```python
from build123d import *
from build123d.topology import SkipClean

# Parameters (mm, degrees)
SKETCH1_W           = 5.06
SKETCH1_H           = 1.900618781
FILLET1_R           = 1
SKETCH2_R           = 7.5
BOSS_EXTRUDE1_DEPTH = 20
SKETCH3_R           = 5.06
CUT_EXTRUDE1_DEPTH  = 5
SKETCH4_R           = 2.5
BOSS_EXTRUDE2_DEPTH = 20
FILLET2_R           = 5
SKETCH6_R           = 0.75
CUT_EXTRUDE2_DEPTH  = 45
FILLET3_R           = 1
FILLET4_R           = 3


# Some blends are built 0.0001 mm under size
with BuildPart() as part:
    # Sketch1 → Revolve1 (revolve)
    with BuildSketch(Plane.XY, mode=Mode.PRIVATE) as revolve1_sk:
        with Locations((-11.747326196, 6.364372648)):
            Rectangle(SKETCH1_W, SKETCH1_H)
        Polygon((-4.277326196, 2.122680798), (-4.277326196, 7.314682038), (-9.217326196, 7.314682038), (-9.217326196, 5.414063257), (-9.217326196, -0.580054764), align=None)
    revolve(revolve1_sk.sketch.rotate(Axis((-14.277326196, 7.314682038, 0), (0, -1, 0)), 90), axis=Axis((-14.277326196, 7.314682038, 0), (0, -1, 0)))

    # Fillet1
    fillet1_edges = [part.edges().sort_by_distance(p)[0] for p in [
        (-14.277326196, -0.580054764, -5.06),
    ]]
    fillet(fillet1_edges, radius=FILLET1_R)

    # Sketch2 → Boss-Extrude1 (add)
    with BuildSketch(Plane(origin=(0, 7.314682038, 0), x_dir=(1, 0, 0), z_dir=(0, 1, 0))):
        with Locations(Location((-14.277326196, 0, 0), (0, 0, 270))):
            Circle(SKETCH2_R)
    extrude(amount=BOSS_EXTRUDE1_DEPTH)

    # Sketch3 → Cut-Extrude1 (cut)
    with BuildSketch(Plane.XZ.offset(-5.414063257)):
        with Locations(Location((-14.277326196, 0, 0), (0, 0, 270))):
            Circle(SKETCH3_R)
    extrude(amount=-CUT_EXTRUDE1_DEPTH, mode=Mode.SUBTRACT)

    # Sketch4 → Boss-Extrude2 (add)
    with BuildSketch(Plane(origin=(0, 27.314682038, 0), x_dir=(1, 0, 0), z_dir=(0, 1, 0))):
        with Locations(Location((-14.277326196, 0, 0), (0, 0, 270))):
            Circle(SKETCH4_R)
    extrude(amount=BOSS_EXTRUDE2_DEPTH)

    # Sketch5 → Revolve2 (revolve)
    with SkipClean():  # the faces are left unmerged after this step: merging them gives an invalid solid
        with BuildSketch(Plane(origin=(0, 47.314682038, 0), x_dir=(1, 0, 0), z_dir=(0, 1, 0))):
            with BuildLine():
                ThreePointArc((-16.777326196, 0), (-14.277326196, 2.5), (-11.777326196, 0))
                Line((-11.777326196, 0), (-6.777326196, 0))
                ThreePointArc((-6.777326196, 0), (-14.277326196, 7.5), (-21.777326196, 0))
                Line((-21.777326196, 0), (-16.777326196, 0))
            make_face()
            with BuildLine():
                Line((-6.777326196, 0), (-11.777326196, 0))
                ThreePointArc((-11.777326196, 0), (-14.277326196, -2.5), (-16.777326196, 0))
                Line((-16.777326196, 0), (-21.777326196, 0))
                ThreePointArc((-21.777326196, 0), (-14.277326196, -7.5), (-6.777326196, 0))
            make_face()
            with BuildLine():
                ThreePointArc((-16.777326196, 0), (-14.277326196, -2.5), (-11.777326196, 0))
                Line((-11.777326196, 0), (-16.777326196, 0))
            make_face()
            with BuildLine():
                Line((-16.777326196, 0), (-11.777326196, 0))
                ThreePointArc((-11.777326196, 0), (-14.277326196, 2.5), (-16.777326196, 0))
            make_face()
        revolve(axis=Axis((-21.777326196, 47.314682038, 0), (1, 0, 0)))
    add(part.part.scale(1), mode=Mode.REPLACE)  # the faces are merged on a copy

    # Fillet2
    fillet2_edges = [part.edges().sort_by_distance(p)[0] for p in [
        (-14.277326196, 27.314682038, -2.5),
    ]]
    fillet(fillet2_edges, radius=FILLET2_R - 0.0001)  # a hair under: the kernel refuses the full size

    # Sketch6 → Cut-Extrude2 (cut)
    with BuildSketch(Plane.XZ.offset(-10.414063257)):
        with Locations(Location((-14.277326196, 0, 0), (0, 0, 270))):
            Circle(SKETCH6_R)
    extrude(amount=-CUT_EXTRUDE2_DEPTH, mode=Mode.SUBTRACT)

    # Fillet3
    fillet3_edges = [part.edges().sort_by_distance(p)[0] for p in [
        (-14.277326196, 54.777087816, 0.749999995),
    ]]
    fillet(fillet3_edges, radius=FILLET3_R)

    # Fillet4
    # the kernel refuses this fillet: 3 mm, written as the material it adds along each edge
    with BuildSketch(Plane(origin=(-14.277326196, 7.314682038, 0), x_dir=(0, 0, 1), z_dir=(-1, 0, 0))) as fillet4_piece_1:
        with BuildLine():
            CenterArc((10.5, 2.958039892), FILLET4_R, 180, 80.405931773)
            Line((10, 0), (9.99, -0.059160798))
            ThreePointArc((9.99, -0.059160798), (8.75, -0.06), (7.5, -0.06))
            Line((7.5, -0.06), (7.44, 0))
            Line((7.44, 0), (7.44, 2.958039892))
            Line((7.44, 2.958039892), (7.5, 2.958039892))
        make_face()
    revolve(axis=Axis((-14.277326196, 7.314682038, 0), (0, 1, 0)))


solid = part.part
```
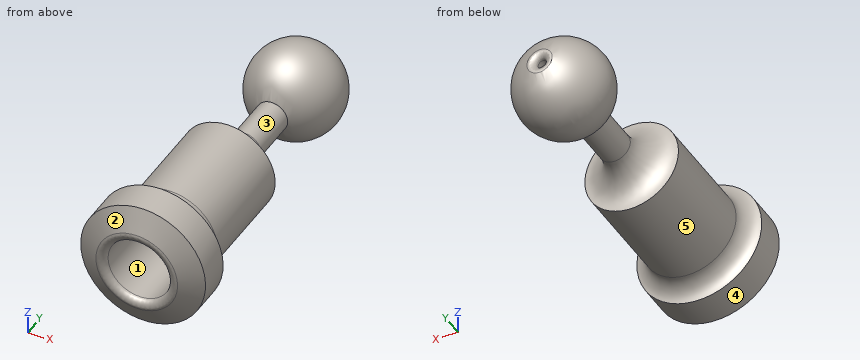
Verification items for the finished model (mm, model axes). Face numbers are marked on the shaded views. A direction names the side the tool comes from. Give positions to 0.01 mm unless a question says otherwise; leave off trailing zeros. Order: outer loops, then holes, each group sorted by start corner. A loop starts at its lowest first (then second) coordinate and runs counter-clockwise, first axis right, second up. Notation, with made-up numbers: (66.5, 68) -> (92.5, 68) arc R34 cw to (92.5, 104) -> close; hole circle Ø1 at (70, 52.5). An arc over 180 degrees is marked (long way). Use a Markdown table: item, result.
1) Section check B-B, the plane y = 36. Record the boundary of the cut face in (x, z), then the cut area to 3 significant figures.
Results:
| item | result |
|---|---|
| outline | circle Ø5 at (-14.28, 0); hole circle Ø1.5 at (-14.28, 0) |
| area | 17.9 mm² |
2) Depth check by flat-ended pin: pin 1 Ø3 at (x, z) = (-17, 1.5) entering from -Y; pin 2 Ø12 at (x, z) = (-18, -2.5) entering from +Y; pin 3 Ø1.5 at (x, z) = (-18.5, 6) entering from -Y; pin 4 Ø10 at (y, z) = (28, -3.5) entering from +X. Enter the tip coordinate at first touch or a pass-through.
Results:
| item | result |
|---|---|
| pin 1 | y = 10.41 |
| pin 2 | y = 54.57 |
| pin 3 | y = 0.26 |
| pin 4 | x = -6.78 |
3) Material ranges on probe 1 along X at (y, z) = (37, 0); probe 2 along Y at (x, z) = (-10, -5); probe 3 along Y at (x, z) = (-8.75, -3.5), recorded low to high.
Results:
| item | result |
|---|---|
| probe 1 | -16.78 to -15.03, -13.53 to -11.78 |
| probe 2 | 0.25 to 27.4, 43.72 to 50.91 |
| probe 3 | 0.23 to 27.41, 43.65 to 50.98 |
4) Section check A-A, the plane y = 4.5. Record the boundary of the cut face in (x, z), then the cut area to 3 significant figures.
Results:
| item | result |
|---|---|
| outline | circle Ø20 at (-14.28, 0); hole circle Ø10.12 at (-14.28, 0) |
| area | 234 mm² |
5) Tool access check on the marked faces 3, 4 and 5. Record the directions out of +Z, -Z, +X, -X, +Y, -Y that give a thin tool (end or side, any length) a straight path to the whole face; none if there is none.
Results:
| item | result |
|---|---|
| face 3 | none |
| face 4 | +Y, -Y |
| face 5 | +Y |
6) Mould release check, pull along X, two halves, no side actions. Record for the marked faces 1 and 2: pulls with the +X half, pulls with the -X half, needs draft (parallel to the pull), parting line crosses it, or undercut.
Results:
| item | result |
|---|---|
| face 1 | undercut |
| face 2 | parting line crosses it |
